Autodesk Inventor part; units mm, degrees
ref_plane "YZ Plane" through (0, 0, 0) normal (1, 0, 0) x (0, 1, 0)
ref_plane "XZ Plane" through (0, 0, 0) normal (0, 1, 0) x (-1, 0, 0)
ref_plane "XY Plane" through (0, 0, 0) normal (0, 0, 1) x (1, 0, 0)
sketch "Sketch1" plane through (0, 0, 0) normal (0, 1, 0) x (-1, 0, 0)
  circle A0 centre (0, 0) radius 7
  circle A1 centre (0, 0) radius 4
  dimension "d0" = 14
  dimension "d1" = 8
extrude "Extrusion1" add sketch "Sketch1" along normal blind 25
sketch "Sketch2" plane through (0, 25, 0) normal (0, 1, 0) x (1, 0, 0)
  circle A0 centre (0, 0) radius 5
  dimension "d4" = 10
extrude "Extrusion2" cut sketch "Sketch2" against normal blind 12.5
sketch "Sketch3" plane through (0, 0, 0) normal (1, 0, 0) x (0, 1, 0)
  circle A0 centre (4, 0) radius 2
  circle A1 centre (21, 0) radius 2
  line L0 (25, -7) -> (25, 7)
  point P0 (0, 0)
  dimension "d7" = 4
  dimension "d8" = 4
  dimension "d9" = 4
  dimension "d10" = 4
extrude "Extrusion3" cut sketch "Sketch3" against normal blind 25
properties part number "Khớp nối cứng"
Geometry check sheet. Reference: the model listing, model coordinates, mm. A direction names the side the tool comes from. Coordinates: 2 decimals unless noted, no trailing zeros. Loops run counter-clockwise (first coordinate to the right, second up) from the corner with the lowest first, then second, coordinate; pieces in that order, holes last.
Item 1: Sectioned sample at A-A, the plane z = 0. Record the boundary of the cut face in (x, y).
Item 2: Sectioned sample at B-B, the plane x = 0. Record the boundary of the cut face in (y, z), then the cut area to 3 significant figures.
Item 3: Sectioned sample at C-C, the plane y = 9.25. Record the boundary of the cut face in (x, z).
Item 4: Sectioned sample at D-D, the plane x = 2.5. Record the boundary of the cut face in (y, z), then the cut area to 3 significant figures.
Item 5: Release check for a two-part mould opening along X. For faces 3 (the face through (2, 25, 5)), 4 (the face through (4.77, 18.84, -1.5)), 5 (the face through (-6.466, 12.325, 2.681)) record: released by +X, released by -X, zero draft, split by the parting line, or undercut.
Item 6: Go/stop test with flat-tipped pins: pin 1 Ø5 at (y, z) = (4, 4) entering from -X; pin 2 Ø4 at (x, y) = (1.5, 18) entering from -Z; pin 3 Ø3 at (y, z) = (21, -3.5) entering from +X; pin 4 Ø2 at (x, y) = (2, 3) entering from -Z. Record where each tip stops, or that it passes through.
Item 7: Thickness scan on line 1 (Y direction, x = -5.5, z = 0); line 2 (Z direction, x = 0, y = 7.25); line 3 (Y direction, x = -4.95, z = 0). Record the ranges inside material, lowest first.
Item 8: Access from +Z, -Z, +X, -X, +Y, -Y to the whole of each face (thin tool, end or side, straight path). Record for faces 1 (the face through (-5.774, 21.923, -1.774)), 2 (the face through (4, 6, 0)).
Check result:
1. outline: (-7, 0) - (-4, 0) - (-4, 2) - (-7, 2) - close; (-7, 6) - (-4, 6) - (-4, 12.5) - (-5, 12.5) - (-5, 19) - (-7, 19) - close; (-7, 23) - (-5, 23) - (-5, 25) - (-7, 25) - close; (4, 0) - (7, 0) - (7, 25) - (5, 25) - (5, 12.5) - (4, 12.5) - close
2. outline: (0, -7) - (25, -7) - (25, -5) - (12.5, -5) - (12.5, -4) - (0, -4) - close; (0, 4) - (12.5, 4) - (12.5, 5) - (25, 5) - (25, 7) - (0, 7) - close
2. area: 125 mm2
3. outline: circle Ø14 at (0, 0); hole circle Ø8 at (0, 0)
4. outline: (0, -6.54) - (25, -6.54) - (25, -4.33) - (12.5, -4.33) - (12.5, -3.12) - (0, -3.12) - close; (0, 3.12) - (12.5, 3.12) - (12.5, 4.33) - (25, 4.33) - (25, 6.54) - (0, 6.54) - close
4. area: 141 mm2
5. face 3: zero draft
5. face 4: undercut
5. face 5: split by the parting line
6. pin 1: stops at x = -6.79
6. pin 2: stops at z = -7
6. pin 3: stops at x = 6.71
6. pin 4: stops at z = -6.93
7. line 1: y = 0 to 2, 6 to 19, 23 to 25
7. line 2: z = -7 to -4, 4 to 7
7. line 3: y = 0 to 2, 6 to 12.5
8. face 1: -X
8. face 2: +Y, -Y
